```python
from build123d import *

# Parameters (mm, degrees)
BOX_W           = 152
BOX_H           = 20
BOX_DEPTH       = 12
SKETCH_R        = 1.7
POCKET_DEPTH    = 20.001
SKETCH001_R     = 4.2
SKETCH001_R_2   = 4.5
SKETCH001_W     = 62
SKETCH001_H     = 8
SKETCH001_H_2   = 9.357648
POCKET001_DEPTH = 12.001
SKETCH002_R     = 8.1
POCKET002_DEPTH = 6.2
SKETCH004_R     = 1.4
POCKET003_DEPTH = 5
SKETCH005_R     = 1.4
POCKET004_DEPTH = 5
SKETCH003_R     = 1.4
POCKET005_DEPTH = 20.001
FILLET_R        = 2.5
FILLET001_R     = 3
FILLET002_R     = 2.8


with BuildPart() as part:
    # Box → Box (new body)
    with BuildSketch(Plane.XY):
        with Locations((76, 10)):
            Rectangle(BOX_W, BOX_H)
    extrude(amount=BOX_DEPTH)

    # Sketch → Pocket (cut, through all)
    with BuildSketch(Plane.XZ):
        with Locations((5, 6)):
            Circle(SKETCH_R)
        with Locations((38, 6)):
            Circle(SKETCH_R)
        with Locations((114, 6)):
            Circle(SKETCH_R)
        with Locations((147, 6)):
            Circle(SKETCH_R)
    extrude(amount=-POCKET_DEPTH, mode=Mode.SUBTRACT)

    # Sketch001 → Pocket001 (cut, through all)
    with BuildSketch(Plane.XY.offset(12)):
        with Locations((12, 7)):
            Circle(SKETCH001_R)
        with Locations((140, 7)):
            Circle(SKETCH001_R)
        with Locations((76, 10)):
            Circle(SKETCH001_R_2)
        with Locations((31, 18)):
            Rectangle(SKETCH001_W, SKETCH001_H)
        with Locations((121, 18.678824)):
            Rectangle(SKETCH001_W, SKETCH001_H_2)
    extrude(amount=-POCKET001_DEPTH, mode=Mode.SUBTRACT)

    # Sketch002 → Pocket002 (cut)
    with BuildSketch(Plane.XY.offset(12)):
        with Locations((76, 10)):
            Circle(SKETCH002_R)
    extrude(amount=-POCKET002_DEPTH, mode=Mode.SUBTRACT)

    # Sketch004 → Pocket003 (cut)
    with BuildSketch(Plane(origin=(0, 14, 0), x_dir=(-1, 0, 0), z_dir=(0, 1, 0))):
        with Locations((-12, 6)):
            Circle(SKETCH004_R)
    extrude(amount=-POCKET003_DEPTH, mode=Mode.SUBTRACT)

    # Sketch005 → Pocket004 (cut)
    with BuildSketch(Plane(origin=(0, 14, 0), x_dir=(-1, 0, 0), z_dir=(0, 1, 0))):
        with Locations((-140, 6)):
            Circle(SKETCH005_R)
    extrude(amount=-POCKET004_DEPTH, mode=Mode.SUBTRACT)

    # Sketch003 → Pocket005 (cut, through all)
    with BuildSketch(Plane(origin=(0, 20, 0), x_dir=(-1, 0, 0), z_dir=(0, 1, 0))):
        with Locations((-76, 8.4)):
            Circle(SKETCH003_R)
    extrude(amount=-POCKET005_DEPTH, mode=Mode.SUBTRACT)

    # Fillet
    fillet_edges = [part.edges().sort_by_distance(p)[0] for p in [
        (152, 14, 6),
        (0, 14, 6),
    ]]
    fillet(fillet_edges, radius=FILLET_R)

    # Fillet001
    fillet001_edges = [part.edges().sort_by_distance(p)[0] for p in [
        (90, 20, 6),
        (62, 20, 6),
    ]]
    fillet(fillet001_edges, radius=FILLET001_R)

    # Fillet002
    fillet002_edges = [part.edges().sort_by_distance(p)[0] for p in [
        (62, 14, 6),
        (90, 14, 6),
    ]]
    fillet(fillet002_edges, radius=FILLET002_R)


solid = part.part
```
The model under review builds one solid part; all positions refer to its coordinate system, in mm. A direction names the side the tool comes from. Round coordinates to 2 decimals unless told otherwise and drop trailing zeros. Loops run counter-clockwise (first coordinate to the right, second up) from the corner with the lowest first, then second, coordinate; pieces in that order, holes last. Notation, with made-up numbers: (79.5, 61.25) -> (98.5, 61.25) arc R23 cw to (98.5, 92.25) -> close; hole circle Ø10 at (-25, -16.5). An arc over 180 degrees is marked (long way). Answer as a JSON object with one key per item and string values. Group by question number.
1) We need section D-D on x = 18.5. Write out the cut boundary in (y, z), then the cut area to 3 significant figures.
2) We need section B-B on x = 147. Write out the cut boundary in (y, z), then the cut area to 3 significant figures.
3) For line 1 (Z direction, x = 5, y = 7.5); line 2 (Z direction, x = 76, y = 18.6); line 3 (Y direction, x = 12, z = 9.75), list the stretches that pass through material, from the lowest coordinate up. Write a range as [from, to].
4) Mouldability with a two-part tool opening along Y and no side actions: class faces 1 (the face through (79.738, 2.814, 8.943)), 2 (the face through (11.09, 2.9, 6.08)), 3 (the face through (151.248, 13.287, 5.916)), 4 (the face through (76.18, 1.03, 9.79)) as released by +Y, released by -Y, zero draft, split by the parting line, or undercut.
5) We need section A-A on y = 7. Write out the cut boundary in (x, z), then the cut area to 3 significant figures.
6) For pin 1 Ø5 at (x, y) = (73, 11) entering from +Z; pin 2 Ø3 at (x, z) = (12, 6) entering from -Y; pin 3 Ø3.5 at (x, z) = (140, 6) entering from +Y, all flat-tipped, find the tip position at first contact; note any pin that passes through.
7) We need section C-C on z = 2.75. Write out the cut boundary in (x, y).
8) For faces 5 (the face through (75, 3, 0)), 6 (the face through (12.18, 12.5, 7.39)), 7 (the face through (79.5, 6.5, 5.8)), 8 (the face through (30, 14, 6)), 9 (the face through (148.57, 6.9, 5.35)), list the 3-axis set-ups (+Z, -Z, +X, -X, +Y, -Y) from which the entire face can be reached by the end or side of a thin tool; tool diameter is ignored.
Result set:
{
 "1": {"outline": "(0, 0) -> (14, 0) -> (14, 12) -> (0, 12) -> close", "area": "168 mm²"},
 "2": {"outline": "(0, 0) -> (14, 0) -> (14, 4.3) -> (0, 4.3) -> close; (0, 7.7) -> (14, 7.7) -> (14, 12) -> (0, 12) -> close", "area": "120 mm²"},
 "3": {"line 1": "[0, 4.3], [7.7, 12]", "line 2": "[0, 7], [9.8, 12]", "line 3": "[0, 2.8], [11.2, 14]"},
 "4": {"face 1": "undercut", "face 2": "undercut", "face 3": "released by +Y", "face 4": "zero draft"},
 "5": {"outline": "(0, 0) -> (7.8, 0) -> (7.8, 12) -> (0, 12) -> close; (16.2, 0) -> (72.65, 0) -> (72.65, 5.8) -> (68.48, 5.8) -> (68.48, 12) -> (16.2, 12) -> close; (79.35, 0) -> (135.8, 0) -> (135.8, 12) -> (83.52, 12) -> (83.52, 5.8) -> (79.35, 5.8) -> close; (144.2, 0) -> (152, 0) -> (152, 12) -> (144.2, 12) -> close; hole circle Ø3.4 at (5, 6); hole circle Ø3.4 at (38, 6); hole circle Ø3.4 at (114, 6); hole circle Ø3.4 at (147, 6)", "area": "1,450 mm²"},
 "6": {"pin 1": "z = 5.8", "pin 2": "y = 0", "pin 3": "y = 14"},
 "7": {"outline": "(0, 0) -> (152, 0) -> (152, 11.5) arc R2.5 ccw to (149.5, 14) -> (92.8, 14) arc R2.8 cw to (90, 16.8) -> (90, 17) arc R3 ccw to (87, 20) -> (65, 20) arc R3 ccw to (62, 17) -> (62, 16.8) arc R2.8 cw to (59.2, 14) -> (2.5, 14) arc R2.5 ccw to (0, 11.5) -> close; hole circle Ø8.4 at (12, 7); hole circle Ø9 at (76, 10); hole circle Ø8.4 at (140, 7)"},
 "8": {"face 5": "-Z, +X, -X, +Y, -Y", "face 6": "+Y", "face 7": "+Z", "face 8": "+Z, -Z, -X, +Y", "face 9": "+Y, -Y"}
}
